```python
from build123d import *

# Parameters (mm, degrees)
BOSS_EXTRUDE2_DEPTH = 20
CUT_EXTRUDE1_DEPTH  = 3
CUT_EXTRUDE2_DEPTH  = 3


with BuildPart() as part:
    # Sketch1 → Boss-Extrude2 (new body)
    with BuildSketch(Plane(origin=(0, 0, 0), x_dir=(0, 0, -1), z_dir=(1, 0, 0))):
        Polygon((0, 0), (0, -28), (28, -28), (28, -25), (3, -25), (3, 0), align=None)
    extrude(amount=-BOSS_EXTRUDE2_DEPTH)

    # Sketch4 → Cut-Extrude1 (cut)
    with BuildSketch(Plane(origin=(0, -25, 0), x_dir=(1, 0, 0), z_dir=(0, 1, 0))):
        with BuildLine():
            Line((-6.5, 17.5), (-6.5, 13.5))
            ThreePointArc((-6.5, 13.5), (-10, 10), (-13.5, 13.5))
            Line((-13.5, 13.5), (-13.5, 17.5))
            ThreePointArc((-13.5, 17.5), (-10, 21), (-6.5, 17.5))
        make_face()
    extrude(amount=-CUT_EXTRUDE1_DEPTH, mode=Mode.SUBTRACT)

    # Sketch5 → Cut-Extrude2 (cut)
    with BuildSketch(Plane(origin=(0, 0, -3), x_dir=(-1, 0, 0), z_dir=(0, 0, -1))):
        with BuildLine():
            Line((13.5, -10.5), (13.5, -14.5))
            ThreePointArc((13.5, -14.5), (10, -18), (6.5, -14.5))
            Line((6.5, -14.5), (6.5, -10.5))
            ThreePointArc((6.5, -10.5), (10, -7), (13.5, -10.5))
        make_face()
    extrude(amount=-CUT_EXTRUDE2_DEPTH, mode=Mode.SUBTRACT)


solid = part.part
```
Part model, mm, in its own coordinate system. A direction names the side the tool comes from. Round coordinates to 2 decimals unless told otherwise and drop trailing zeros. Loops run counter-clockwise (first coordinate to the right, second up) from the corner with the lowest first, then second, coordinate; pieces in that order, holes last.
1. Slice it at A-A (y = -13.25). Give the cut face in (x, z), and give its area (3 significant figures).
Solutions:
outline: (-20, -3) - (-13.5, -3) - (-13.5, 0) - (-20, 0) - close; (-6.5, -3) - (0, -3) - (0, 0) - (-6.5, 0) - close
area: 39.0 mm2
2. Flat gauge pins, fed straight in: pin 1 (0.9 mm diameter, centred on y = -12.5, z = -2, fed in from +X); pin 2 (1.5 mm diameter, centred on x = -12.5, z = -8, fed in from +Y). Where does each tip first touch, or does it go through?
Solutions:
pin 1: stops at x = 0
pin 2: stops at y = -25
3. 3-axis set-ups, long thin cutter, end or side, ignore diameter. For faces 1 (the face through (-5, -13, -3)), 2 (the face through (-10, -7, -2)), 3 (the face through (-10, -26, -21)): which of +Z, -Z, +X, -X, +Y, -Y reach the whole face in a straight line?
Solutions:
face 1: -Z, +X, -X, +Y
face 2: +Z, -Z
face 3: +Y, -Y
4. Slice it at B-B (x = -10). Give the cut face in (y, z).
Solutions:
outline: (-28, -28) - (-25, -28) - (-25, -21) - (-28, -21) - close; (-28, -10) - (-25, -10) - (-25, -3) - (-18, -3) - (-18, 0) - (-28, 0) - close; (-7, -3) - (0, -3) - (0, 0) - (-7, 0) - close
5. Two-plate mould, pull along Y, no slides. Class faces 4 (the face through (-7.6, -28, -10.7)), 5 (the face through (-10, -26, -10)), 6 (the face through (-6.5, -13, -2)): pulls with the +Y half, pulls with the -Y half, needs draft (parallel to the pull), parting line crosses it, or undercut.
Solutions:
face 4: pulls with the -Y half
face 5: needs draft
face 6: undercut
6. Drill centre lines: line 1 along Y through (x, z) = (-16.25, -4.25); line 2 along Z through (x, y) = (-17.75, -2.25). Where is each one in solid material? Low to high.
Solutions:
line 1: y = -28 to -25
line 2: z = -3 to 0
7. Slice it at D-D (x = -7.5). Give the cut face in (y, z).
Solutions:
outline: (-28, -28) - (-25, -28) - (-25, -19.95) - (-28, -19.95) - close; (-28, -11.05) - (-25, -11.05) - (-25, -3) - (-16.95, -3) - (-16.95, 0) - (-28, 0) - close; (-8.05, -3) - (0, -3) - (0, 0) - (-8.05, 0) - close
8. Slice it at C-C (z = -18). Give the cut face in (x, y), and give its area (3 significant figures).
Solutions:
outline: (-20, -28) - (-13.46, -28) - (-13.46, -25) - (-20, -25) - close; (-6.54, -28) - (0, -28) - (0, -25) - (-6.54, -25) - close
area: 39.2 mm2
